CAD build for the part. Positions are in the model's coordinates, mm. Round coordinates to 2 decimals unless told otherwise and drop trailing zeros. Write each loop counter-clockwise with the first axis right and the second up, starting at its lowest first coordinate (ties: lowest second). Pieces come first, ordered by that corner, then holes. Notation, with made-up numbers: (9.5, 69) - (24.5, 69) arc R15 cw to (24.5, 87) - close; hole circle Ø6 at (18.25, -14). An arc over 180 degrees is marked (long way). Use one line per item in the form item = value. Start each with the question number.
Item 1: Drill centre lines: L1, parallel to X at y = -4.5, z = -15; L2, parallel to X at y = -13, z = -9.5; L3, parallel to X at y = 12, z = 11. Where is each one in solid material? Low to high.
Item 2: Band-saw the part on A-A, the plane x = 1147.5. List the corners of the cut face in (y, z), and give its area (3 significant figures).
Item 3: Pin check, flat tips, straight feed: pin 1 (2 mm diameter, centred on y = 13, z = 11.5, fed in from +X); pin 2 (5 mm diameter, centred on y = 1, z = 15.5, fed in from +X); pin 3 (1 mm diameter, centred on y = 7.5, z = -10, fed in from +X); pin 4 (12 mm diameter, centred on y = 10.5, z = -8.5, fed in from -X). Stop position of each tip, or through.
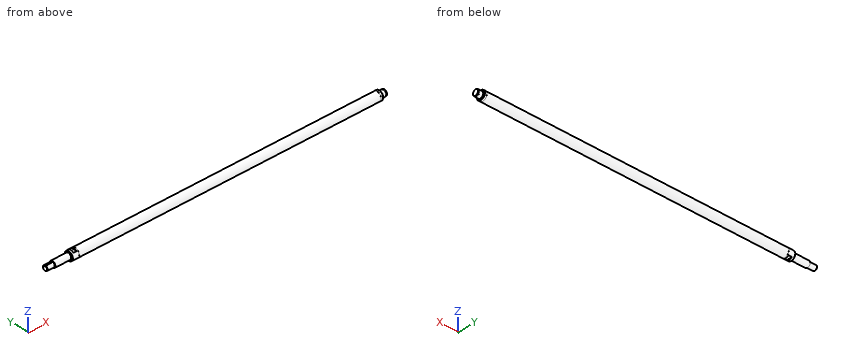
from build123d import *

# Parameters (mm, degrees)
SKETCH1_W          = 1229
SKETCH1_H          = 18
SKETCH3_W          = 13
SKETCH3_H          = 36
CUT_EXTRUDE1_DEPTH = 9
SKETCH4_W          = 13
SKETCH4_H          = 36
CUT_EXTRUDE2_DEPTH = 9
CUT_EXTRUDE3_DEPTH = 3.5


with BuildPart() as part:
    # Sketch1 → Revolve1 (revolve)
    with BuildSketch(Plane.XY, mode=Mode.PRIVATE) as revolve1_sk:
        with Locations((619.5, 9)):
            Rectangle(SKETCH1_W, SKETCH1_H)
    revolve(revolve1_sk.sketch.rotate(Axis((1234, 0, 0), (-1, 0, 0)), 180), axis=Axis((1234, 0, 0), (-1, 0, 0)))

    # Sketch2 → Revolve2 (revolve)
    with BuildSketch(Plane.XY, mode=Mode.PRIVATE) as revolve2_sk:
        Polygon((-118, 0), (-118, 8.888888889), (-116.888888889, 10), (-88, 10), (-88, 11.58), (-87.08, 12.5), (-23, 12.5), (-23, 16.2), (-21.2, 18), (4.8, 18), (4.8, 14.4), (5, 14.4), (5, 0), align=None)
    revolve(revolve2_sk.sketch.rotate(Axis((5, 0, 0), (-1, 0, 0)), 180), axis=Axis((5, 0, 0), (-1, 0, 0)))

    # Sketch3 → Cut-Extrude1 (cut)
    with BuildSketch(Plane.XY.offset(13.5)):
        with Locations((-6.5, 0)):
            Rectangle(SKETCH3_W, SKETCH3_H)
    extrude(amount=CUT_EXTRUDE1_DEPTH, mode=Mode.SUBTRACT)

    # Sketch4 → Cut-Extrude2 (cut)
    with BuildSketch(Plane.XY.offset(-13.5)):
        with Locations((-6.5, 0)):
            Rectangle(SKETCH4_W, SKETCH4_H)
    extrude(amount=-CUT_EXTRUDE2_DEPTH, mode=Mode.SUBTRACT)

    # Sketch5 → Cut-Extrude3 (cut)
    with BuildSketch(Plane.XY.offset(10)):
        with BuildLine():
            Line((-118, -3), (-96, -3))
            ThreePointArc((-96, -3), (-93, 0), (-96, 3))
            Line((-96, 3), (-118, 3))
            Line((-118, 3), (-118, -3))
        make_face()
    extrude(amount=-CUT_EXTRUDE3_DEPTH, mode=Mode.SUBTRACT)

    # Sketch6 → Revolve3 (revolve)
    with BuildSketch(Plane.XY, mode=Mode.PRIVATE) as revolve3_sk:
        Polygon((1234, 0), (1234, 14.4), (1234.2, 14.4), (1234.2, 18), (1242.2, 18), (1244, 16.2), (1244, 12.5), (1259, 12.5), (1259, 11.95), (1260.35, 11.95), (1260.35, 12.5), (1262.75, 12.5), (1264, 11.25), (1264, 0), align=None)
    revolve(revolve3_sk.sketch.rotate(Axis((1264, 0, 0), (-1, 0, 0)), 180), axis=Axis((1264, 0, 0), (-1, 0, 0)))


solid = part.part
Determined:
q1.L1 = -23 to -13, 0 to 4.8, 5 to 1234, 1234.2 to 1244
q1.L2 = -23 to 4.8, 5 to 1234, 1234.2 to 1244
q1.L3 = -22.92 to 4.8, 5 to 1234, 1234.2 to 1243.92
q2.outline = circle Ø36 at (0, 0)
q2.area = 1,020 mm²
q3.pin_1 = 1243.84
q3.pin_2 = 1244
q3.pin_3 = 1263.25
q3.pin_4 = -118
